```python
from build123d import *

# Parameters (mm, degrees)
CYLINDER013_R     = 8
CYLINDER013_DEPTH = 110
CYLINDER015_R     = 9.8
CYLINDER015_DEPTH = 110
CHAMFER_SIZE      = 1


with BuildPart() as negative:
    # Cylinder013 → Cylinder013 (new body)
    with BuildSketch(Plane.XY.offset(2)):
        Circle(CYLINDER013_R)
    extrude(amount=CYLINDER013_DEPTH)


with BuildPart() as central_tube:
    # Cylinder015 → Cylinder015 (new body)
    with BuildSketch(Plane.XY):
        Circle(CYLINDER015_R)
    extrude(amount=CYLINDER015_DEPTH)

    # Cut: cut negative
    add(negative.part, mode=Mode.SUBTRACT)

    # Chamfer
    chamfer_edges = [central_tube.edges().sort_by_distance(p)[0] for p in [
        (-9.8, 0, 0),
    ]]
    chamfer(chamfer_edges, length=CHAMFER_SIZE)


solid = central_tube.part
```
Source: CAD feature listing. Evaluate the final solid. Frame: model axes, mm. A direction names the side the tool comes from. Give positions to 0.01 mm unless a question says otherwise; leave off trailing zeros. Write each loop counter-clockwise with the first axis right and the second up, starting at its lowest first coordinate (ties: lowest second). Pieces come first, ordered by that corner, then holes.
1. First-contact query: pin 1 (1.5 mm diameter, centred on x = -1, z = 77, fed in from -Y). Flat tip, straight axial feed; report the tip coordinate or a pass-through.
2. Pull-direction query (Y, two-part tool) for faces 3 (the face through (-1.73, -7.81, 55.24)), 4 (the face through (-2.124, -9.567, 54.737)), 5 (the face through (-8.03, 1.5, 110)); classes: +Y half, -Y half, draft (parallel to the pull), parting line (faces both ways), or undercut.
3. Section query C-C (z = 82.5). Return the cut outline in (x, y), then the cut area to 3 significant figures.
4. Access query for faces 1 (the face through (0, 0, 2)), 2 (the face through (0, 0, 0)). Directions: +Z, -Z, +X, -X, +Y, -Y. A direction counts if a zero-diameter tool reaches every point of the face in a straight line with its end or side. Return the directions, or none.
5. Material intervals for line 1 along Y through (x, z) = (0, 24); line 2 along Z through (x, y) = (-1.75, 3); line 3 along Y through (x, z) = (6.75, 43), sorted ascending.
6. Section query A-A (y = 0). Return the cut outline in (x, z), then the cut area to 3 significant figures.
Output values:
1. pin 1: stops at y = -9.8
2. face 3: undercut
2. face 4: parting line
2. face 5: draft
3. outline: circle Ø19.6 at (0, 0); hole circle Ø16 at (0, 0)
3. area: 101 mm2
4. face 1: +Z
4. face 2: -Z, +X, -X, +Y, -Y
5. line 1: y = -9.8 to -8, 8 to 9.8
5. line 2: z = 0 to 2
5. line 3: y = -7.1 to -4.29, 4.29 to 7.1
6. outline: (-9.8, 1) - (-8.8, 0) - (8.8, 0) - (9.8, 1) - (9.8, 110) - (8, 110) - (8, 2) - (-8, 2) - (-8, 110) - (-9.8, 110) - close
6. area: 427 mm2
